```python
from build123d import *

# Parameters (mm, degrees)
SKETCH1_W           = 69.85
SKETCH1_H           = 21.59
BOSS_EXTRUDE1_DEPTH = 5.08
SKETCH2_W           = 25.019
SKETCH2_H           = 15.494
SKETCH2_W_2         = 18.669
SKETCH2_H_2         = 9.144
BOSS_EXTRUDE2_DEPTH = 10.16
FILLET2_R           = 1.905
FILLET3_R           = 1.27


with BuildPart() as part:
    # Sketch1 → Boss-Extrude1 (new body)
    with BuildSketch(Plane.XY):
        Rectangle(SKETCH1_W, SKETCH1_H)
    extrude(amount=BOSS_EXTRUDE1_DEPTH)

    # Sketch2 → Boss-Extrude2 (add)
    with BuildSketch(Plane.XY.offset(5.08)):
        Rectangle(SKETCH2_W, SKETCH2_H)
        Rectangle(SKETCH2_W_2, SKETCH2_H_2, mode=Mode.SUBTRACT)
    extrude(amount=BOSS_EXTRUDE2_DEPTH)

    # Fillet2
    fillet2_edges = [part.edges().sort_by_distance(p)[0] for p in [
        (12.5095, -7.747, 10.16),
        (12.5095, 7.747, 10.16),
        (-12.5095, 7.747, 10.16),
        (-12.5095, -7.747, 10.16),
        (34.925, -10.795, 2.54),
        (-34.925, -10.795, 2.54),
        (-34.925, 10.795, 2.54),
        (34.925, 10.795, 2.54),
    ]]
    fillet(fillet2_edges, radius=FILLET2_R)

    # Fillet3
    fillet3_edges = [part.edges().sort_by_distance(p)[0] for p in [
        (-12.5095, 0, 5.08),
        (0, 7.747, 5.08),
        (12.5095, 0, 5.08),
        (0, -7.747, 5.08),
        (-11.951538418, 7.189038418, 5.08),
        (11.951538418, 7.189038418, 5.08),
        (11.951538418, -7.189038418, 5.08),
        (-11.951538418, -7.189038418, 5.08),
    ]]
    fillet(fillet3_edges, radius=FILLET3_R)


solid = part.part
```
For this review, take the finished solid that the model builds, in its own axes (mm). A direction names the side the tool comes from. Coordinates: 2 decimals unless noted, no trailing zeros. Loops run counter-clockwise (first coordinate to the right, second up) from the corner with the lowest first, then second, coordinate; pieces in that order, holes last. Notation, with made-up numbers: (-2, 31) - (41, 31) arc R31 ccw to (41, 60) - close; hole circle Ø3 at (57.25, 8.5). An arc over 180 degrees is marked (long way). Use one line per item in the form item = value. Start each with the question number.
1) Take a section at B-B (x = 10). State the section outline as (y, z) points (3 decimals), plus the area to 3 significant figures.
2) Take a section at D-D (x = 20). State the section outline as (y, z) points (3 decimals).
3) Take a section at A-A (z = 8.5). State the section outline as (x, y) points (1 decimal), plus the area to 3 significant figures.
4) Draft analysis for pull direction Y (two halves, no side actions). For faces 1 (the face through (-34.382, -10.222, 2.576)), 2 (the face through (0, -4.572, 10)), 3 (the face through (-34.382, 10.222, 2.576)), state which applies: released by +Y, released by -Y, zero draft, split by the parting line, or undercut.
5) To check wall thickness, follow probe 1 along Y at (x, z) = (4, 8.25); probe 2 along X at (y, z) = (-4, 6.5); probe 3 along Z at (x, y) = (-28, 5.5). State the ranges of each line that lie inside material, in increasing order. Write a range as from..to.
6) For pin 1 (10 mm diameter, centred on x = -26.5, y = -7.5, fed in from -Z); pin 2 (4.5 mm diameter, centred on y = 3, z = 12, fed in from +X); pin 3 (1 mm diameter, centred on x = -20.5, y = 7, fed in from +Z); pin 4 (3 mm diameter, centred on x = -1, z = 10, fed in from +Y), all flat-tipped, find the tip position at first contact; note any pin that passes through.
7) For faces 4 (the face through (11.94, -7.2, 10.86)), 5 (the face through (12.51, 0, 11)), 6 (the face through (0, -7.747, 11)), 7 (the face through (9.334, 0, 10)), list the 3-axis set-ups (+Z, -Z, +X, -X, +Y, -Y) from which the entire face can be reached by the end or side of a thin tool; tool diameter is ignored.
From the geometry:
q1.outline = (-10.795, 0) - (10.795, 0) - (10.795, 5.08) - (9.017, 5.08) arc R1.27 cw to (7.747, 6.35) - (7.747, 15.24) - (-7.747, 15.24) - (-7.747, 6.35) arc R1.27 cw to (-9.017, 5.08) - (-10.795, 5.08) - close
q1.area = 268 mm2
q2.outline = (-10.795, 0) - (10.795, 0) - (10.795, 5.08) - (-10.795, 5.08) - close
q3.outline = (-12.5, -5.8) arc R1.9 ccw to (-10.6, -7.7) - (10.6, -7.7) arc R1.9 ccw to (12.5, -5.8) - (12.5, 5.8) arc R1.9 ccw to (10.6, 7.7) - (-10.6, 7.7) arc R1.9 ccw to (-12.5, 5.8) - close; hole (-9.3, -4.6) - (9.3, -4.6) - (9.3, 4.6) - (-9.3, 4.6) - close
q3.area = 214 mm2
q4.face_1 = released by -Y
q4.face_2 = undercut
q4.face_3 = released by +Y
q5.probe_1 = -7.75..-4.57, 4.57..7.75
q5.probe_2 = -12.51..-9.33, 9.33..12.51
q5.probe_3 = 0..5.08
q6.pin_1 = 0
q6.pin_2 = 12.51
q6.pin_3 = 5.08
q6.pin_4 = 7.75
q7.face_4 = +Z, +X, -Y
q7.face_5 = +Z, +X, +Y, -Y
q7.face_6 = +Z, +X, -X, -Y
q7.face_7 = +Z
